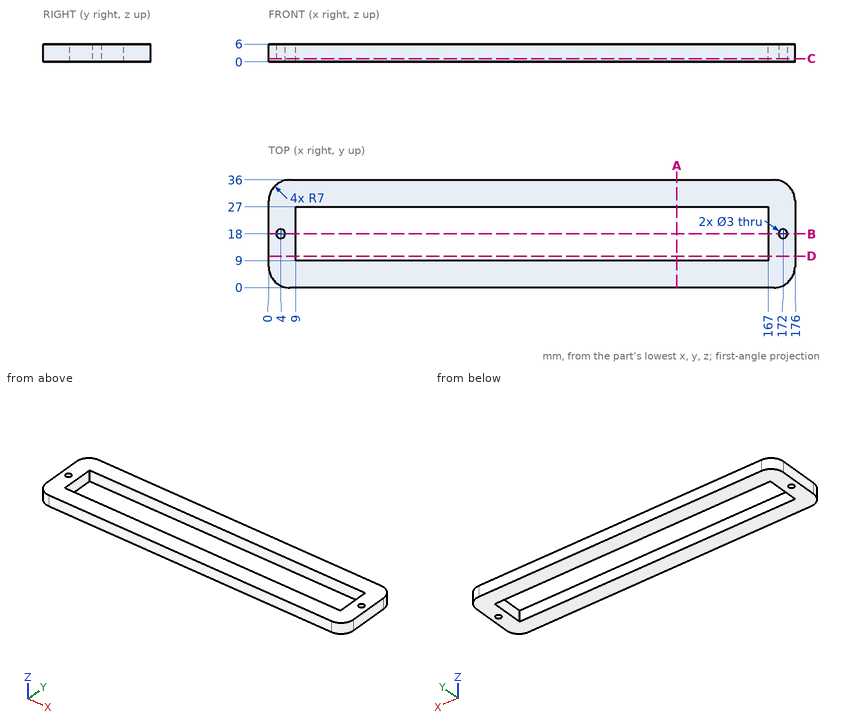
The drawing under review shows one solid part. Ordinate dimensions are in mm from its lowest x, y, z. Give positions to 0.01 mm unless a question says otherwise; leave off trailing zeros. Write each loop counter-clockwise with the first axis right and the second up, starting at its lowest first coordinate (ties: lowest second). Pieces come first, ordered by that corner, then holes.
1. Add section C-C, the plane z = 1.1. Write out the cut boundary in (x, y), plus the area to 3 significant figures.
2. Add section A-A, the plane x = 136.5. Write out the cut boundary in (y, z), plus the area to 3 significant figures.
3. Add section B-B, the plane y = 18. Write out the cut boundary in (x, z), plus the area to 3 significant figures.
4. For P1, Ø1, axis at y = 5.5, z = 5, coming from the -X side; P2, Ø3, axis at x = 69.5, y = 7, coming from the -Z side; P3, Ø2, axis at y = 32, z = 5, coming from the +X side, all flat-tipped, find the tip position at first contact; note any pin that passes through.
5. Wall thickness on L1, parallel to Y at x = 160.5, z = 1.2; L2, parallel to X at y = 20, z = 5.6; L3, parallel to Y at x = 172, z = 1.5: over which ranges is each line inside the solid? List them lowest first.
6. Add section D-D, the plane y = 10.5. Write out the cut boundary in (x, z).
Worked answers:
1. outline: (0, 7) arc R7 ccw to (7, 0) - (169, 0) arc R7 ccw to (176, 7) - (176, 29) arc R7 ccw to (169, 36) - (7, 36) arc R7 ccw to (0, 29) - close; hole circle Ø3 at (4, 18); hole (9, 9) - (167, 9) - (167, 27) - (9, 27) - close; hole circle Ø3 at (172, 18)
1. area: 3,440 mm2
2. outline: (0, 0) - (9, 0) - (9, 6) - (0, 6) - close; (27, 0) - (36, 0) - (36, 6) - (27, 6) - close
2. area: 108 mm2
3. outline: (0, 0) - (2.5, 0) - (2.5, 6) - (0, 6) - close; (5.5, 0) - (9, 0) - (9, 6) - (5.5, 6) - close; (167, 0) - (170.5, 0) - (170.5, 6) - (167, 6) - close; (173.5, 0) - (176, 0) - (176, 6) - (173.5, 6) - close
3. area: 72.0 mm2
4. P1: stops at x = 0.07
4. P2: stops at z = 0
4. P3: stops at x = 175.71
5. L1: y = 0 to 9, 27 to 36
5. L2: x = 0 to 9, 167 to 176
5. L3: y = 0.68 to 16.5, 19.5 to 35.32
6. outline: (0, 0) - (9, 0) - (9, 6) - (0, 6) - close; (167, 0) - (176, 0) - (176, 6) - (167, 6) - close
